from build123d import *

# Parameters (mm, degrees)
SKETCH1_R           = 10
BOSS_EXTRUDE1_DEPTH = 13
SKETCH2_R           = 14
BOSS_EXTRUDE2_DEPTH = 19
SKETCH3_R           = 11
CUT_EXTRUDE1_DEPTH  = 6
SKETCH4_R           = 9
CUT_EXTRUDE2_DEPTH  = 10
SKETCH5_R           = 5
CUT_EXTRUDE3_DEPTH  = 33
FILLET1_R           = 0.05


with BuildPart() as part:
    # Sketch1 → Boss-Extrude1 (new body)
    with BuildSketch(Plane(origin=(0, 0, 0), x_dir=(0, 0, -1), z_dir=(1, 0, 0))):
        Circle(SKETCH1_R)
    extrude(amount=BOSS_EXTRUDE1_DEPTH)

    # Sketch2 → Boss-Extrude2 (add)
    with BuildSketch(Plane.ZY):
        Circle(SKETCH2_R)
    extrude(amount=BOSS_EXTRUDE2_DEPTH)

    # Sketch3 → Cut-Extrude1 (cut)
    with BuildSketch(Plane.ZY.offset(19)):
        Circle(SKETCH3_R)
    extrude(amount=-CUT_EXTRUDE1_DEPTH, mode=Mode.SUBTRACT)

    # Sketch4 → Cut-Extrude2 (cut)
    with BuildSketch(Plane.ZY.offset(13)):
        Circle(SKETCH4_R)
    extrude(amount=-CUT_EXTRUDE2_DEPTH, mode=Mode.SUBTRACT)

    # Sketch5 → Cut-Extrude3 (cut, through all)
    with BuildSketch(Plane(origin=(13, 0, 0), x_dir=(0, 0, -1), z_dir=(1, 0, 0))):
        Circle(SKETCH5_R)
    extrude(amount=-CUT_EXTRUDE3_DEPTH, mode=Mode.SUBTRACT)

    # Fillet1
    fillet1_edges = [part.edges().sort_by_distance(p)[0] for p in [
        (-19, 0, -11),
    ]]
    fillet(fillet1_edges, radius=FILLET1_R)


solid = part.part
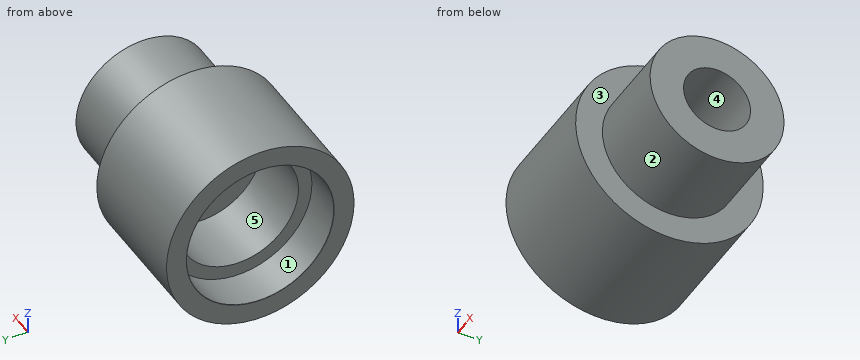
Work out the finished part from the listing and answer in its coordinate system (mm). Face numbers are marked on the shaded views. A direction names the side the tool comes from. Coordinates: 2 decimals unless noted, no trailing zeros. Write each loop counter-clockwise with the first axis right and the second up, starting at its lowest first coordinate (ties: lowest second). Pieces come first, ordered by that corner, then holes. Notation, with made-up numbers: M 63.25,-4.5 L 85.25,-4.5 A18 ccw 85.25,12.5 Z; hole C -16,74.5 d4. An arc over 180 degrees is marked long. Use one line per item in the form item = value. Start each with the question number.
1. The part is cut by section A-A (z = 0). Give the vertices of the cut face in (x, y), plus the area to 3 significant figures.
2. The part is cut by section C-C (x = -3.5). Give the vertices of the cut face in (y, z).
3. The mould has two halves that part along Y. Classify the marked faces 1, 2 and 3: released by +Y, released by -Y, zero draft, split by the parting line, or undercut.
4. The part is cut by section D-D (x = 5.5). Give the vertices of the cut face in (y, z), plus the area to 3 significant figures.
5. Each of these flat-tipped pins is pushed along its axis until it touches: P1, Ø1.5, axis at x = -10.5, y = 4, coming from the +Z side; P2, Ø12, axis at x = 7, y = 7, coming from the -Z side; P3, Ø9, axis at y = 0, z = 0, coming from the -X side; P4, Ø11, axis at y = 1.5, z = -4.5, coming from the -X side. Where does it stop, or does it pass through?
6. A tool of negligible diameter and unlimited length cuts with its end or side. For the marked faces 4 and 5, from which of +Z, -Z, +X, -X, +Y, -Y can it reach the whole face along a straight path? Write none if from no direction.
7. Straight lines are drawn through the part: probe 1 along Y at (x, z) = (4.25, 0); probe 2 along Y at (x, z) = (-15.35, 0); probe 3 along X at (y, z) = (-1.5, 7.25). For each, find the intervals that lie inside material, in ascending order. Write a range as from..to.
Evaluation:
q1.outline = M -19,-14 L 0,-14 L 0,-10 L 13,-10 L 13,-5 L -3,-5 L -3,-9 L -13,-9 L -13,-11 L -18.95,-11 A0.05 ccw -19,-11.05 Z; M -19,11.05 A0.05 ccw -18.95,11 L -13,11 L -13,9 L -3,9 L -3,5 L 13,5 L 13,10 L 0,10 L 0,14 L -19,14 Z
q1.area = 320 mm^2
q2.outline = C 0,0 d28; hole C 0,0 d18
q3.face_1 = undercut
q3.face_2 = split by the parting line
q3.face_3 = zero draft
q4.outline = C 0,0 d20; hole C 0,0 d10
q4.area = 236 mm^2
q5.P1 = 13.62
q5.P2 = -9.95
q5.P3 = through
q5.P4 = -13
q6.face_4 = +X, -X
q6.face_5 = -X
q7.probe_1 = -10..-5, 5..10
q7.probe_2 = -14..-11, 11..14
q7.probe_3 = -3..13
